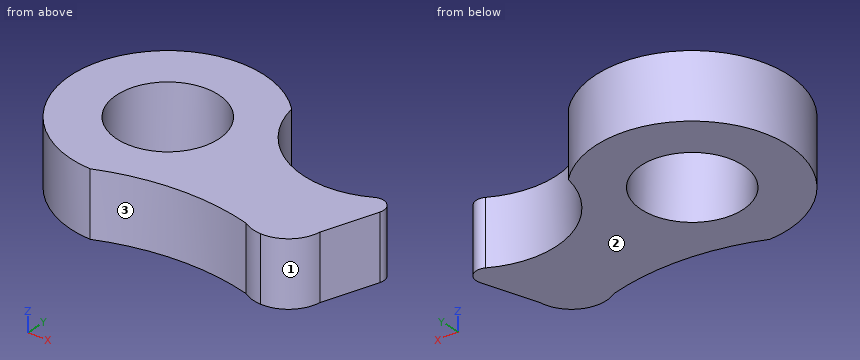
```python
from build123d import *

# Parameters (mm, degrees)
F0_R     = 20.091447
F1_DEPTH = 25.4


with BuildPart() as f1:
    # F0 (on Top) → F1 (new body)
    with BuildSketch(Plane.XY):
        with BuildLine():
            ThreePointArc((78.119229, 3.16254), (46.20116, 1.853494), (26.713748, 27.165892))
            ThreePointArc((26.713748, 27.165892), (-35.260676, 14.43242), (0, -38.1))
            ThreePointArc((0, -38.1), (27.921411, -30.791494), (56.714284, -32.78896))
            ThreePointArc((56.714284, -32.78896), (60.321561, -33.720822), (63.88674, -34.802633))
            ThreePointArc((63.88674, -34.802633), (73.027903, -31.334338), (77.567758, -22.67526))
            Line((77.567758, -22.67526), (84.701062, -2.319822))
            ThreePointArc((84.701062, -2.319822), (83.312466, 2.705184), (78.119229, 3.16254))
        make_face()
        Circle(F0_R, mode=Mode.SUBTRACT)
        with BuildLine():
            ThreePointArc((63.88674, -34.802633), (60.321561, -33.720822), (56.714284, -32.78896))
            ThreePointArc((56.714284, -32.78896), (60.161857, -34.289667), (63.88674, -34.802633))
        make_face()
    extrude(amount=F1_DEPTH)


solid = f1.part
```
Model file for the job. Use its own axes, mm. Face numbers are marked on the shaded views. Coordinates: 2 decimals unless noted, no trailing zeros. Loops run counter-clockwise (first coordinate to the right, second up) from the corner with the lowest first, then second, coordinate; pieces in that order, holes last. Notation, with made-up numbers: (-32.5, 2.25) - (-7.5, 2.25) arc R32 cw to (-7.5, 39.25) - close; hole circle Ø1 at (29.5, 12). An arc over 180 degrees is marked (long way). Answer as a JSON object with one key per item and string values. Group by question number.
(1) Flat gauge pins, fed straight in: pin 1 (3 mm diameter, centred on y = 25.5, z = 6, fed in from +X); pin 2 (12 mm diameter, centred on y = 22.5, z = 7, fed in from -X); pin 3 (3 mm diameter, centred on x = -17, y = -1, fed in from +Z) (3 decimals); pin 4 (1.5 mm diameter, centred on x = 50.5, z = 4.5, fed in from -Y). Where does each tip first touch, or does it go through?
(2) Cut at C-C (y = -11.5). Give the cut face in (x, z), then the cut area to 3 significant figures.
(3) Probe line 1 along Y through (x, z) = (0, 9); line 2 along X through (y, z) = (14.5, 9.75); line 3 along X through (y, z) = (-3, 15.25). List the from-to ranges inside material, lowest first.
(4) Cut at D-D (z = 2). Give the cut face in (x, y), then the cut area to 3 significant figures.
(5) Cut at A-A (x = -4). Give the cut face in (y, z).
(6) Two-plate mould, pull along X, no slides. Class the marked faces 1, 2 and 3: released by +X, released by -X, zero draft, split by the parting line, or undercut.
(7) Cut at B-B (y = 0). Give the cut face in (x, z), then the cut area to 3 significant figures.
Geometry says:
{
 "1": {"pin 1": "stops at x = 27.44", "pin 2": "stops at x = -34.34", "pin 3": "passes through", "pin 4": "stops at y = -31.68"},
 "2": {"outline": "(-36.32, 0) - (-16.47, 0) - (-16.47, 25.4) - (-36.32, 25.4) - close; (16.47, 0) - (81.48, 0) - (81.48, 25.4) - (16.47, 25.4) - close", "area": "2,160 mm^2"},
 "3": {"line 1": "y = -38.1 to -20.09, 20.09 to 38.1", "line 2": "x = -35.23 to -13.91, 13.91 to 31.71", "line 3": "x = -37.98 to -19.87, 19.87 to 84.46"},
 "4": {"outline": "(0, -38.1) arc R89.12 cw to (56.71, -32.79) arc R13.78 ccw to (63.89, -34.8) arc R13.78 ccw to (77.57, -22.68) - (84.7, -2.32) arc R4.57 ccw to (78.12, 3.16) arc R34.73 cw to (26.71, 27.17) arc R38.1 ccw (long way) to start; hole circle Ø40.18 at (0, 0)", "area": "4,760 mm^2"},
 "5": {"outline": "(-37.89, 0) - (-19.69, 0) - (-19.69, 25.4) - (-37.89, 25.4) - close; (19.69, 0) - (37.89, 0) - (37.89, 25.4) - (19.69, 25.4) - close"},
 "6": {"face 1": "released by +X", "face 2": "zero draft", "face 3": "undercut"},
 "7": {"outline": "(-38.1, 0) - (-20.09, 0) - (-20.09, 25.4) - (-38.1, 25.4) - close; (20.09, 0) - (51.11, 0) - (51.11, 25.4) - (20.09, 25.4) - close; (70.69, 0) - (84.89, 0) - (84.89, 25.4) - (70.69, 25.4) - close", "area": "1,610 mm^2"}
}
